Autodesk Inventor part; units mm, degrees
ref_plane "YZ Plane" through (0, 0, 0) normal (1, 0, 0) x (0, 1, 0)
ref_plane "XZ Plane" through (0, 0, 0) normal (0, 1, 0) x (-1, 0, 0)
ref_plane "XY Plane" through (0, 0, 0) normal (0, 0, 1) x (1, 0, 0)
sketch "Skizze1" plane through (0, 0, 0) normal (0, 0, 1) x (1, 0, 0)
  line L0 (0, 0) -> (42, 0)
  line L1 (0, 0) -> (0, 15)
  line L2 (0, 15) -> (14, 15)
  line L3 (14, 15) -> (14, 9)
  line L4 (14, 9) -> (19, 9)
  line L5 (19, 9) -> (20, 10)
  line L6 (20, 10) -> (33, 10)
  line L7 (33, 10) -> (34, 9)
  line L8 (34, 9) -> (42, 9)
  line L9 (42, 9) -> (42, 0)
  dimension "d0" = 45
  dimension "d1" = 42
  dimension "d2" = 20
  dimension "d3" = 18
  dimension "d4" = 5
  dimension "d5" = 28
  dimension "d6" = 8
  dimension "d7" = 30
revolve "Umdrehung1" add sketch "Skizze1" angle 360 about axis through (0, 0, 0) along (1, 0, 0)
thread "Gewinde1"
sketch "Skizze2" plane through (0, 0, 0) normal (-1, 0, 0) x (0, 0, 1)
  circle A0 centre (0, 0) radius 15
hole "Bohrung1" at (0, 0, 0) direction (1, 0, 0) diameter 14 depth 42
sketch "Skizze3" plane through (0, 0, 0) normal (-1, 0, 0) x (0, 0, 1)
  circle A0 centre (0, 0) radius 15
  line L0 (9, 12) -> (-9, 12)
  circle A1 centre (0, 0) radius 15
  line L1 (9, -12) -> (-9, -12)
  line L2 (15, 0) -> (-15, 0) construction
  point P0 (-9, -12)
  point P1 (-9, 12)
  dimension "d18" = 24
extrude "Extrusion1" cut sketch "Skizze3" against normal up to surface (14 mm away) contours L0 A0 | A0 L1
fillet "Rundung1" radius 2 1 edges at (14, -9, 0)
properties part number "Arbeitszylinder" material "Titan"
Design review of the part built by this model. Coordinates are the model's own, in mm. A direction names the side the tool comes from. Round coordinates to 2 decimals unless told otherwise and drop trailing zeros. Write each loop counter-clockwise with the first axis right and the second up, starting at its lowest first coordinate (ties: lowest second). Pieces come first, ordered by that corner, then holes. Notation, with made-up numbers: (-18, -1) -> (23, -1) arc R34 cw to (23, 30) -> close; hole circle Ø4 at (72.5, 20). An arc over 180 degrees is marked (long way). Write item = value, one per line. Start each with the question number.
1) Take a section at D-D, the plane x = 15.5. State the section outline as (y, z) points, plus the area to 3 significant figures.
2) Clearance check with flat-ended pins moving along their axes: pin 1 (1 mm diameter, centred on x = 11, y = -9, fed in from -Z); pin 2 (8 mm diameter, centred on x = 30, z = 3.5, fed in from -Y); pin 3 (8 mm diameter, centred on x = 17, y = -3.5, fed in from -Z). State where each tip first meets the part, or that it passes through.
3) Tool access review of faces 1 (the face through (38.056, -1.172, 8.923)), 2 (the face through (17.521, -1.172, 8.923)), 3 (the face through (7, -12, 0)): name each direction out of +Z, -Z, +X, -X, +Y, -Y from which nothing blocks a thin tool from reaching the whole face with its end or side.
4) Take a section at A-A, the plane z = 0. State the section outline as (x, y) points, plus the area to 3 significant figures.
5) Take a section at C-C, the plane x = 36. State the section outline as (y, z) points, plus the area to 3 significant figures.
6) Take a section at B-B, the plane y = 0. State the section outline as (x, z) points.
7) Mouldability with a two-part tool opening along Y and no side actions: class faces 4 (the face through (0, -3, 7)), 5 (the face through (7, 0, -15)), 6 (the face through (7, 12, 0)), 7 (the face through (21.294, 2.681, 6.466)) as +Y half, -Y half, draft (parallel to the pull), parting line (faces both ways), or undercut.
8) Wall thickness on probe 1 along Z at (x, y) = (17, 0); probe 2 along Y at (x, z) = (9, 0); probe 3 along Z at (x, y) = (23.5, 0): over which ranges is each line inside the solid? List them lowest first. Write a range as from..to.
Results list:
q1.outline = circle Ø18.13 at (0, 0); hole circle Ø14 at (0, 0)
q1.area = 104 mm²
q2.pin_1 = -12.36
q2.pin_2 = -10
q2.pin_3 = -14.98
q3.face_1 = +X
q3.face_2 = none
q3.face_3 = +Z, -Z, +X, -X, -Y
q4.outline = (0, -12) -> (14, -12) -> (14, -11) arc R2 cw to (16, -9) -> (19, -9) -> (20, -10) -> (33, -10) -> (34, -9) -> (42, -9) -> (42, -7) -> (0, -7) -> close; (0, 7) -> (42, 7) -> (42, 9) -> (34, 9) -> (33, 10) -> (20, 10) -> (19, 9) -> (16, 9) arc R2 cw to (14, 11) -> (14, 12) -> (0, 12) -> close
q4.area = 282 mm²
q5.outline = circle Ø18 at (0, 0); hole circle Ø14 at (0, 0)
q5.area = 101 mm²
q6.outline = (0, -15) -> (14, -15) -> (14, -11) arc R2 cw to (16, -9) -> (19, -9) -> (20, -10) -> (33, -10) -> (34, -9) -> (42, -9) -> (42, -7) -> (0, -7) -> close; (0, 7) -> (42, 7) -> (42, 9) -> (34, 9) -> (33, 10) -> (20, 10) -> (19, 9) -> (16, 9) arc R2 cw to (14, 11) -> (14, 15) -> (0, 15) -> close
q7.face_4 = draft
q7.face_5 = parting line
q7.face_6 = +Y half
q7.face_7 = undercut
q8.probe_1 = -9..-7, 7..9
q8.probe_2 = -12..-7, 7..12
q8.probe_3 = -10..-7, 7..10
